Geometry check sheet. Reference: drawing and pictorial views, mm from the part's lowest x, y, z. Coordinates: 2 decimals unless noted, no trailing zeros. Loops run counter-clockwise (first coordinate to the right, second up) from the corner with the lowest first, then second, coordinate; pieces in that order, holes last. Notation, with made-up numbers: (36.25, -4) - (83.25, -4) arc R28 ccw to (83.25, 26) - close; hole circle Ø7 at (17.5, 8.5). An arc over 180 degrees is marked (long way). One line per item, written item: value.
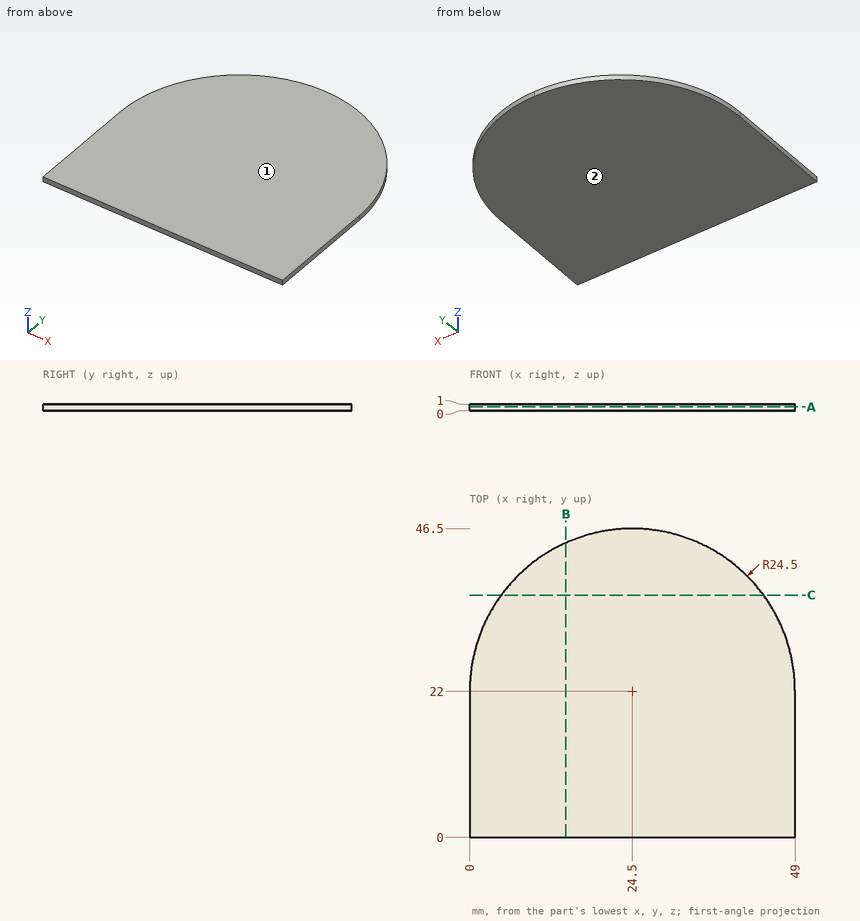
(1) Release check for a two-part mould opening along Z. For the marked faces 1 and 2 record: pulls with the +Z half, pulls with the -Z half, needs draft (parallel to the pull), parting line crosses it, or undercut.
Reply:
face 1: pulls with the +Z half
face 2: pulls with the -Z half
(2) Cross-section at A-A on z = 0.55. Record the cut outline in (x, y), and give its area (3 significant figures).
Reply:
outline: (0, 0) - (49, 0) - (49, 22) arc R24.5 ccw to (0, 22) - close
area: 2,020 mm2
(3) Cross-section at C-C on y = 36.5. Record the cut outline in (x, z), and give its area (3 significant figures).
Reply:
outline: (4.75, 0) - (44.25, 0) - (44.25, 1) - (4.75, 1) - close
area: 39.5 mm2
(4) Cross-section at B-B on x = 14.5. Record the cut outline in (y, z), and give its area (3 significant figures).
Reply:
outline: (0, 0) - (44.37, 0) - (44.37, 1) - (0, 1) - close
area: 44.4 mm2
(5) Material ranges on probe 1 along X at (y, z) = (29, 0.5); probe 2 along X at (y, z) = (41, 0.5); probe 3 along Y at (x, z) = (10, 0.55), recorded low to high. Write a range as from..to.
Reply:
probe 1: 1.02..47.98
probe 2: 9.03..39.97
probe 3: 0..41.75
